Autodesk Inventor part; units mm, degrees
ref_plane "Work Plane1" through (30, 0, 0) normal (0, -0.5, 0.866) x (1, 0, 0)
ref_plane "YZ Plane" through (0, 0, 0) normal (1, 0, 0) x (0, 1, 0)
ref_plane "XZ Plane" through (0, 0, 0) normal (0, 1, 0) x (-1, 0, 0)
sketch "Эскиз1" plane through (0, 0, 0) normal (0, 0, 1) x (1, 0, 0)
  line L0 (-0.19, 0) -> (8, 0)
  line L1 (8, 0) -> (8, 2.5)
  line L2 (8, 2.5) -> (1.6, 2.5)
  line L3 (1.6, 2.5) -> (1.1092, 2.5)
  line L4 (1.1092, 2.5) -> (0, 2.5)
  line L5 (0, 2.5) -> (0, 4.75)
  line L6 (0, 4.75) -> (-2.75, 4.75)
  line L7 (-2.75, 4.75) -> (-2.75, 1.7321)
  line L8 (-2.75, 1.7321) -> (-1.19, 1.7321)
  line L9 (-1.19, 1.7321) -> (-0.19, 0)
  line L10 (-4.9, 0) -> (10.15, 0)
  line L11 (0, -0.95) -> (0, 5.7)
  line L12 (1.6, 2.5) -> (0, 2.5) construction
  dimension "d0" = 6.4
  dimension "d1" = 0.4908
  dimension "d2" = 2.75
  dimension "d3" = 1.56
  dimension "d4" = 60
  dimension "d5" = 5
  dimension "d6" = 5
  dimension "d7" = 3.4641
  dimension "d8" = 9.5
  dimension "d19" = 8
revolve "Базовый элемент" add sketch "Эскиз1" angle 360 about axis through (-0.19, 0, 0) along (1, 0, 0)
sketch "Эскиз2" plane through (-2.75, 0, 0) normal (-1, 0, 0) x (0, 0, 1)
  circle A0 centre (0, 0) radius 1.7321
  line L0 (0, -6.65) -> (0, 6.65)
  line L1 (-6.65, 0) -> (6.65, 0)
  line L2 (1.7321, 0) -> (0.866, -1.5)
  line L3 (0.866, -1.5) -> (-0.866, -1.5)
  line L4 (-0.866, -1.5) -> (-1.7321, 0)
  line L5 (-1.7321, 0) -> (-0.866, 1.5)
  line L6 (-0.866, 1.5) -> (0.866, 1.5)
  line L7 (0.866, 1.5) -> (1.7321, 0)
extrude "Паз" add sketch "Эскиз2" against normal up to next contours L7 A0 | A0 L2 | L6 L0 A0 | A0 L0 L3 | L0 L6 A0 | A0 L3 L0 | L4 A0 | A0 L5
fillet "Сопряжение1" radius 2.375 1 edges at (-2.75, -4.75, 0)
thread "Резьба"
chamfer "Фаска1" distance 0.4908 distance2 0.4908 1 edges at (8, -2.5, 0) measured on face at (8, -0.6238, -0.819)
fillet "Сопряжение2" radius 0.2 1 edges at (0, -2.5, 0)
ref_plane "Work Plane1" through (30, 0, 0) normal (0, -0.5, 0.866) x (1, 0, 0)
equation "\"d0\" = GEL"
equation "\"d1\" = GAL"
equation "\"d2\" = KOH"
equation "\"d3\" = INTI"
equation "\"d5\" = GD"
equation "\"d6\" = BDM"
equation "\"d7\" = 1.1547 * SW"
equation "\"d8\" = KOD"
equation "\"d19\" = NLG"
equation "\"d16\" = RR"
equation "\"d12\" = GEL"
equation "\"d14\" = -0.5 * SPD + 0.5 * GD"
equation "\"d15\" = GUL"
equation "\"d29\" = R"
equation "\"GD\" = NND"
equation "\"NLG\" = 8"
equation "\"GEL\" = 6.4"
equation "\"KOD\" = 9.5"
equation "\"KOH\" = 2.75"
equation "\"INTI\" = 1.56"
equation "\"GAL\" = 0.61345 * PTC"
equation "\"GUL\" = 0.61345 * PTC"
equation "\"BDM\" = NND"
equation "\"SW\" = 3"
equation "\"RR\" = 2.375"
equation "\"SPD\" = 4.01848"
equation "\"d28\" = R"
equation "\"R\" = 0.2"
equation "\"TOA\" = 30deg"
equation "\"THREADDIA\" = 5"
equation "\"KOD1\" = KOD - 2 * RR"
equation "\"PTC\" = 0.8"
equation "\"NND\" = 5"
equation "\"E0\" = 1.155 * SW"
equation "\"GD1\" = THREADDIA - 1.2269 * PTC"
properties part number "ANSI B18.3.4M - M5 x 0.8 x 8, BHSBHCSM" material "Сталь, мягкая"
The model under review builds one solid part; all positions refer to its coordinate system, in mm. A direction names the side the tool comes from. Give positions to 0.01 mm unless a question says otherwise; leave off trailing zeros. Write each loop counter-clockwise with the first axis right and the second up, starting at its lowest first coordinate (ties: lowest second). Pieces come first, ordered by that corner, then holes.
1. Wall thickness on L1, parallel to Z at x = -1, y = 0.5; L2, parallel to Z at x = -2, y = -0.25; L3, parallel to X at y = -2.75, z = -1: over which ranges is each line inside the solid? List them lowest first.
2. For P1, Ø1.4, axis at x = -2, z = 0, coming from the -Y side; P2, Ø1.9, axis at x = -2, z = 0, coming from the +Y side; P3, Ø1.5, axis at x = 6, z = 3.5, coming from the +Y side, all flat-tipped, find the tip position at first contact; note any pin that passes through.
3. Add section A-A, the plane x = 5.5. Write out the cut boundary in (y, z).
4. Tool access review of faces 4 (the flat face through (8, 0, 0)), 5 (the flat face through (-2, 1.5, 0)): name each direction out of +Z, -Z, +X, -X, +Y, -Y from which nothing blocks a thin tool from reaching the whole face with its end or side.
5. Draft analysis for pull direction Y (two halves, no side actions). For faces 1 (the flat face through (0, 2.04, -2.04)), 2 (the flat face through (-2, -1.5, 0)), 3 (the cylindrical face through (3.8, -0.54, 2.44)), state which applies: +Y half, -Y half, draft (parallel to the pull), parting line (faces both ways), or undercut.
Worked answers:
1. L1: z = -4.64 to -1.31, 1.31 to 4.64
1. L2: z = -4.1 to -1.59, 1.59 to 4.1
1. L3: x = -2.69 to 0
2. P1: stops at y = -4.56
2. P2: stops at y = 4.65
2. P3: passes through
3. outline: circle Ø5 at (0, 0)
4. face 4: +Z, -Z, +X, +Y, -Y
4. face 5: -X
5. face 1: draft
5. face 2: undercut
5. face 3: parting line
